CAD build for the part. Positions are in the model's coordinates, mm. Coordinates: 2 decimals unless noted, no trailing zeros. Loops run counter-clockwise (first coordinate to the right, second up) from the corner with the lowest first, then second, coordinate; pieces in that order, holes last. Notation, with made-up numbers: (46, 24.5) -> (57, 24.5) arc R23 ccw to (57, 33.5) -> close; hole circle Ø5 at (-16.75, 41.25). An arc over 180 degrees is marked (long way). Write item = value, one per line. Start each with the question number.
(1) Band-saw the part on B-B (x = 33.5). Write the cut outline in (y, z), and give its area (3 significant figures).
(2) Band-saw the part on C-C (y = -38). Write the cut outline in (x, z), and give its area (3 significant figures).
(3) Band-saw the part on A-A (z = 38). Write the cut outline in (x, y).
(4) Flat gauge pins, fed straight in: P1, Ø6, axis at y = -22.5, z = 7, coming from the +X side; P2, Ø1, axis at x = 31.5, z = 26.5, coming from the +Y side; P3, Ø8, axis at x = 65, y = -7.5, coming from the +Z side. Where does each tip first touch, or does it go through?
(5) Drill centre lines: line 1 (Z direction, x = 12, y = -1); line 2 (X direction, y = -13, z = 40); line 3 (X direction, y = 15, z = 26). Where is each one in solid material? Low to high. Write a range as from..to.
```python
from build123d import *

# Parameters (mm, degrees)
F1_DEPTH = 33
F2_DEPTH = 44
F4_DEPTH = 66.001


with BuildPart() as f1:
    # F0 (on Front) → F1 (new body, symmetric)
    with BuildSketch(Plane.XZ):
        Polygon((77, 0), (0, 66), (0, 51.512144), (60.097502, 0), align=None)
    extrude(amount=F1_DEPTH, both=True)

    # F0 (on Front) → F2 (join, symmetric)
    with BuildSketch(Plane.XZ):
        Polygon((77, 0), (0, 66), (0, 51.512144), (60.097502, 0), align=None)
    extrude(amount=F2_DEPTH, both=True)

    # F3 (on Top) → F4 (intersect, through all)
    with BuildSketch(Plane.XY):
        Polygon((88.684835, -51.202213), (88.684835, 51.202213), (0, 0), align=None)
    extrude(amount=F4_DEPTH, mode=Mode.INTERSECT)


solid = f1.part
```
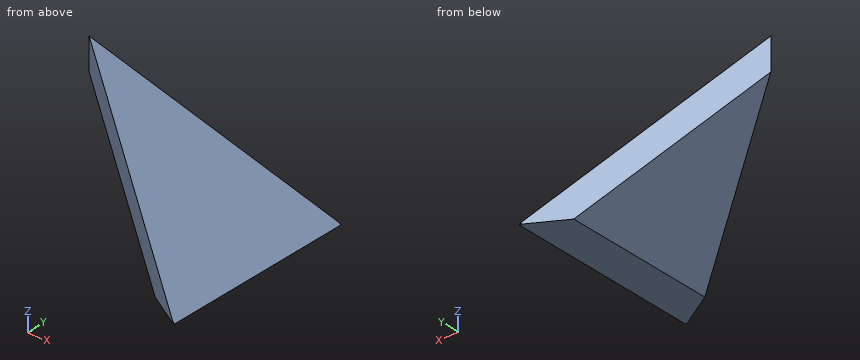
Findings below:
q1.outline = (-19.34, 22.8) -> (19.34, 22.8) -> (19.34, 37.29) -> (-19.34, 37.29) -> close
q1.area = 560 mm²
q2.outline = (65.82, 0) -> (77, 0) -> (65.82, 9.58) -> close
q2.area = 53.6 mm²
q3.outline = (15.76, -9.1) -> (32.67, -18.86) -> (32.67, 18.86) -> (15.76, 9.1) -> close
q4.P1 = 72.33
q4.P2 = 18.48
q4.P3 = 13.71
q5.line_1 = 41.23..55.71
q5.line_2 = 22.52..30.33
q5.line_3 = 29.76..46.67
